Geometry: final body of the model. Coordinates: model frame, mm. Face numbers are marked on the shaded views. A direction names the side the tool comes from. Round coordinates to 2 decimals unless told otherwise and drop trailing zeros. Loops run counter-clockwise (first coordinate to the right, second up) from the corner with the lowest first, then second, coordinate; pieces in that order, holes last. Notation, with made-up numbers: (59, 53) - (106, 53) arc R14 ccw to (106, 63) - close; hole circle Ø11 at (-24.5, 85.5). An arc over 180 degrees is marked (long way). Write item = value, one per line. Start each with the question number.
Item 1: Draft query along X for the marked faces 3, 4 and 5. Return one class per face: pulls with the +X half, pulls with the -X half, needs draft (parallel to the pull), parting line crosses it, or undercut.
Item 2: First-contact query: pin 1 (2 mm diameter, centred on y = 7, z = 30, fed in from +X); pin 2 (1.5 mm diameter, centred on x = -17.5, z = 30, fed in from -Y); pin 3 (2 mm diameter, centred on x = -16.5, z = 29.5, fed in from +Y). Flat tips, straight axial feed; report the tip coordinate or a pass-through.
Item 3: Section B-B (z = 30.4). Return loops of the section in (x, y).
Item 4: Section C-C (x = -15.25). Return loops of the section in (y, z).
Item 5: Access query for the marked faces 1 and 2. Directions: +Z, -Z, +X, -X, +Y, -Y. A direction counts if a zero-diameter tool reaches every point of the face in a straight line with its end or side. Return the directions, or none.
Item 6: Line query: line 1 (Y direction, x = -14.25, z = 29.8); line 2 (Z direction, x = -16, y = -20.5); line 3 (X direction, y = -4, z = 28.5). Output: solid intervals per line, ascending. Write a range as from..to.
Item 7: Section D-D (y = -6). Return loops of the section in (x, z).
from build123d import *

# Parameters (mm, degrees)
F0_W     = 9
F0_H     = 4
F1_DEPTH = 25
F2_W     = 4.6
F2_H     = 4
F3_DEPTH = 4.2
F4_R     = 1.3
F5_DEPTH = 25
F6_R     = 1.99999


# Not quite as in the source:
# - a fillet or chamfer is up to 0.001 mm smaller than in the source, because OpenCascade refuses the exact size


with BuildPart() as f1:
    # F0 (on Front) → F1 (new body)
    with BuildSketch(Plane.XZ):
        with Locations((-22.8743378759, 29.5677930117)):
            Rectangle(F0_W, F0_H)
    extrude(amount=F1_DEPTH)

    # F2 (on face) → F3 (join)
    with BuildSketch(Plane.YZ.offset(-18.3743378759)):
        with Locations((-20.5, 29.5677930117)):
            Rectangle(F2_W, F2_H)
    extrude(amount=F3_DEPTH)

    # F4 (on face) → F5 (cut)
    with BuildSketch(Plane.XZ.offset(22.8)):
        with Locations((-15.9743378759, 29.5677930117)):
            Circle(F4_R)
    extrude(amount=-F5_DEPTH, mode=Mode.SUBTRACT)

    # F6 (radius 2 in the source; OpenCascade refuses exactly that, so slightly less here)
    f6_edges = [f1.edges().sort_by_distance(p)[0] for p in [
        (-14.174338, -20.5, 31.567793),
        (-14.174338, -20.5, 27.567793),
    ]]
    fillet(f6_edges, radius=F6_R)

    # F7: F1 across face


with BuildPart() as f1_1:
    add(f1.part)
    add(f1.part.mirror(Plane(origin=(-22.8743378759, 0, 29.5677930117), x_dir=(1, 0, 0), z_dir=(0, 1, 0))))


with BuildPart() as f8_1:
    # F8: copy of F1
    add(f1_1.part)


solid = f1_1.part
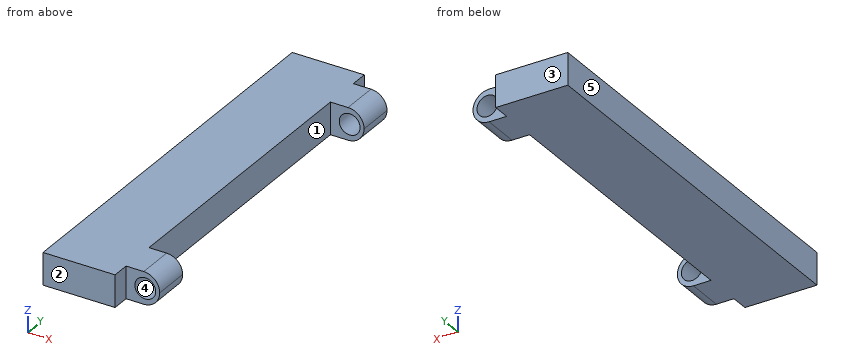
Taken from the geometry:
q1.face_3 = needs draft
q1.face_4 = undercut
q1.face_5 = pulls with the -X half
q2.pin_1 = -18.37
q2.pin_2 = -22.8
q2.pin_3 = 22.8
q3.outline = (-27.37, -25) - (-18.37, -25) - (-18.37, -22.8) - (-16.97, -22.8) - (-16.97, -18.2) - (-18.37, -18.2) - (-18.37, 18.2) - (-16.97, 18.2) - (-16.97, 22.8) - (-18.37, 22.8) - (-18.37, 25) - (-27.37, 25) - close; (-14.98, -22.8) - (-14.36, -22.8) - (-14.36, -18.2) - (-14.98, -18.2) - close; (-14.98, 18.2) - (-14.36, 18.2) - (-14.36, 22.8) - (-14.98, 22.8) - close
q4.outline = (-22.8, 27.79) - (-18.2, 27.79) - (-18.2, 28.49) - (-22.8, 28.49) - close; (-22.8, 30.65) - (-18.2, 30.65) - (-18.2, 31.34) - (-22.8, 31.34) - close; (18.2, 27.79) - (22.8, 27.79) - (22.8, 28.49) - (18.2, 28.49) - close; (18.2, 30.65) - (22.8, 30.65) - (22.8, 31.34) - (18.2, 31.34) - close
q5.face_1 = +Z, -Z, +X
q5.face_2 = +Z, -Z, +X, -X, -Y
q6.line_1 = -22.8..-18.2, 18.2..22.8
q6.line_2 = 27.58..28.27, 30.87..31.56
q6.line_3 = -27.37..-18.37
q7.outline = (-27.37, 27.57) - (-18.37, 27.57) - (-18.37, 31.57) - (-27.37, 31.57) - close
